For this review, take the finished solid that the model builds, in its own axes (mm). A direction names the side the tool comes from. Give positions to 0.01 mm unless a question says otherwise; leave off trailing zeros. Order: outer loops, then holes, each group sorted by start corner. A loop starts at its lowest first (then second) coordinate and runs counter-clockwise, first axis right, second up. Notation, with made-up numbers: (28.5, -24) - (64.5, -24) arc R12 cw to (64.5, -11) - close; hole circle Ø1 at (63.5, 52). An arc over 180 degrees is marked (long way). One line per item, written item: value.
```python
from build123d import *

# Parameters (mm, degrees)
SALIENTE_EXTRUIR1_DEPTH = 3
REVOLUCI_N1_ANGLE       = 180
SALIENTE_EXTRUIR2_DEPTH = 3
CROQUIS4_R              = 1.6
CORTAR_EXTRUIR1_DEPTH   = 3
SALIENTE_EXTRUIR3_START = 15
CROQUIS5_R              = 6
CROQUIS5_R_2            = 1.6
SALIENTE_EXTRUIR3_DEPTH = 15


with BuildPart() as part:
    # Croquis1 → Saliente-Extruir1 (new body)
    with BuildSketch(Plane.XY):
        with BuildLine():
            Line((-80.787332882, 3.645984144), (-50.787332882, 3.645984144))
            ThreePointArc((-50.787332882, 3.645984144), (-65.787332882, 18.645984144), (-80.787332882, 3.645984144))
        make_face()
    extrude(amount=SALIENTE_EXTRUIR1_DEPTH)

    # Croquis2 → Revolución1 (revolve)
    with BuildSketch(Plane.XZ.offset(-3.645984144)):
        with BuildLine():
            Line((-65.787332882, 18), (-65.787332882, 16.2))
            ThreePointArc((-65.787332882, 16.2), (-75.121142393, 12.333809512), (-78.987332882, 3))
            Line((-78.987332882, 3), (-80.787332882, 3))
            ThreePointArc((-80.787332882, 3), (-76.393934599, 13.606601718), (-65.787332882, 18))
        make_face()
    revolve(axis=Axis((-65.787332882, 3.645984144, 3), (0, 0, -1)), revolution_arc=REVOLUCI_N1_ANGLE)

    # Croquis3 → Saliente-Extruir2 (add)
    with BuildSketch(Plane(origin=(0, 0, 0), x_dir=(-1, 0, 0), z_dir=(0, 0, -1))):
        with BuildLine():
            Line((65.787332882, 3.645984144), (71.787332882, 3.645984144))
            ThreePointArc((71.787332882, 3.645984144), (65.787332882, -2.354015856), (59.787332882, 3.645984144))
            Line((59.787332882, 3.645984144), (65.787332882, 3.645984144))
        make_face()
    extrude(amount=-SALIENTE_EXTRUIR2_DEPTH)

    # Croquis4 → Cortar-Extruir1 (cut)
    with BuildSketch(Plane(origin=(0, 0, 0), x_dir=(-1, 0, 0), z_dir=(0, 0, -1))):
        with Locations((65.787332882, 3.645984144)):
            Circle(CROQUIS4_R)
    extrude(amount=-CORTAR_EXTRUIR1_DEPTH, mode=Mode.SUBTRACT)

    # Croquis5 → Saliente-Extruir3 (add)
    with BuildSketch(Plane(origin=(0, 0, 0), x_dir=(-1, 0, 0), z_dir=(0, 0, -1)).offset(SALIENTE_EXTRUIR3_START)):
        with Locations((65.787332882, 3.645984144)):
            Circle(CROQUIS5_R)
        with Locations((65.787332882, 3.645984144)):
            Circle(CROQUIS5_R_2, mode=Mode.SUBTRACT)
    extrude(amount=-SALIENTE_EXTRUIR3_DEPTH)


solid = part.part
```
(1) Take a section at D-D (x = -78.25). Write out the cut boundary in (y, z).
Answers below:
outline: (3.65, 0) - (11.99, 0) - (11.99, 3) arc R8.35 ccw to (3.65, 11.35) - (3.65, 7.35) arc R4.35 cw to (8, 3) - (3.65, 3) - close
(2) Draft analysis for pull direction Y (two halves, no side actions). For faces 1 (the face through (-66.8, 3.646, 16.4)), 2 (the face through (-64.19, 3.72, -6.13)), 3 (the face through (-66, 7, 3)), 4 (the face through (-65.457, 18.642, 1.479)), state which applies: pulls with the +Y half, pulls with the -Y half, needs draft (parallel to the pull), parting line crosses it, or undercut.
Answers below:
face 1: pulls with the -Y half
face 2: undercut
face 3: needs draft
face 4: pulls with the +Y half
(3) Machinability: for faces 5 (the face through (-64.487, -2.211, -6.126)), 6 (the face through (-66, 11, 0)), 7 (the face through (-67, 2, -15)), which of the approach directions +Z, -Z, +X, -X, +Y, -Y give a long, thin tool a straight path to every point of the face, cutting with its end or side? Answer none if there is none.
Answers below:
face 5: -Z
face 6: -Z, +Y
face 7: -Z, +X, -X, +Y, -Y
(4) For P1, Ø3, axis at x = -72.5, y = 3.5, coming from the +Z side; P2, Ø5, axis at y = 1, z = 1.5, coming from the +X side; P3, Ø10, axis at x = -69.5, z = -5.5, coming from the +Y side; P4, Ø1, axis at x = -58, y = 1.5, coming from the +Z side (1 decimal), all flat-tipped, find the tip position at first contact; note any pin that passes through.
Answers below:
P1: stops at z = 17.06
P2: stops at x = -59.79
P3: stops at y = 9.65
P4: passes through
(5) Wall thickness on line 1 (X direction, y = 3.75, z = -9); line 2 (Z direction, x = -64.25, y = -1); line 3 (Z direction, x = -57, y = 7.5): over which ranges is each line inside the solid? List them lowest first. Write a range as from..to.
Answers below:
line 1: x = -71.79..-67.38, -64.19..-59.79
line 2: z = -15..3
line 3: z = 0..3, 12.06..14.53
(6) Take a section at B-B (z = 2.5). Write out the cut boundary in (x, y), then the cut area to 3 significant figures.
Answers below:
outline: (-80.79, 3.65) - (-71.79, 3.65) arc R6 ccw to (-59.79, 3.65) - (-50.79, 3.65) arc R15 ccw to start; hole circle Ø3.2 at (-65.79, 3.65)
area: 402 mm^2
(7) Take a section at A-A (y = 2.75). Write out the cut boundary in (x, z).
Answers below:
outline: (-71.72, -15) - (-67.11, -15) - (-67.11, 3) - (-71.72, 3) - close; (-64.46, -15) - (-59.85, -15) - (-59.85, 3) - (-64.46, 3) - close
